Autodesk Inventor part; units mm, degrees
ref_plane "YZ Plane" through (0, 0, 0) normal (1, 0, 0) x (0, 1, 0)
ref_plane "XZ Plane" through (0, 0, 0) normal (0, 1, 0) x (-1, 0, 0)
ref_plane "XY Plane" through (0, 0, 0) normal (0, 0, 1) x (1, 0, 0)
sketch "Sketch1" plane through (0, 0, 0) normal (0, 0, 1) x (1, 0, 0)
  circle A0 centre (0, 0) radius 4
  arc A1 (-6, 0) -> (6, 0) centre (0, 0) ccw
  line L0 (0, 21) -> (13.5, 21)
  line L1 (13.5, 21) -> (-13.5, 21)
  line L2 (-13.5, 21) -> (-13.5, 12)
  line L3 (-13.5, 12) -> (-6, 0)
  line L4 (13.5, 21) -> (13.5, 12)
  line L5 (13.5, 12) -> (6, 0)
  dimension "d0" = 8
  dimension "d1" = 12
  dimension "d2" = 21
  dimension "d3" = 13.5
  dimension "d4" = 27
  dimension "d5" = 9
  dimension "d6" = 9
extrude "Extrusion1" add sketch "Sketch1" along normal blind 3
sketch "Sketch2" plane through (13.5, 12, 0) normal (1, 0, 0) x (0, 0, -1)
  line L0 (8, 20) -> (-3, 9)
  line L1 (8, 20) -> (68, 20)
  line L2 (79, 9) -> (68, 20)
  line L3 (0, 9) -> (-3, 9)
  line L4 (-3, 9) -> (0, 9)
  line L5 (0, 9) -> (8, 17)
  line L6 (79.1439, 8.8561) -> (76.1439, 8.8561)
  line L7 (76.1439, 8.8561) -> (68, 17)
  line L8 (39.224, 17) -> (8, 17)
  line L9 (39.224, 17) -> (68, 17)
  line L10 (-3, 0) -> (-3, -12)
  line L11 (8, 17) -> (68, 17)
  line L12 (-3, 9) -> (0, 9)
  line L13 (0, 9) -> (8, 17)
  line L14 (8, 17) -> (68, 17)
  line L15 (76.1439, 8.8561) -> (79.1439, 8.8561)
  line L16 (79.1439, 8.8561) -> (68, 20)
  line L17 (68, 20) -> (8, 20)
  line L18 (8, 20) -> (-3, 9)
  line L19 (-3, 9) -> (0, 9)
  point P0 (0, -12)
  dimension "d11" = 60
  dimension "d14" = 3
extrude "Extrusion2" add sketch "Sketch2" against normal blind 27
sketch "Sketch3" plane through (13.5, 20.8561, -79.1439) normal (0, -1, 0) x (1, 0, 0)
  line L0 (0, 0) -> (-27, 0)
  line L1 (0, 0) -> (-27, 0)
  line L2 (0, 3) -> (-27, 3)
  line L3 (-27, 0) -> (-27, 3)
  line L4 (-27, 3) -> (0, 3)
  line L5 (0, 3) -> (0, 0)
  point P0 (-13.5, 79.1439)
extrude "Extrusion3" add sketch "Sketch3" along normal blind 45
sketch "Sketch4" plane through (13.5, 29, -68) normal (0, -1, 0) x (1, 0, 0)
  line L0 (0, 0) -> (0, 60)
  line L1 (0, 1.254) -> (-27, 1.254)
  line L2 (-27, 0) -> (-27, 60)
  line L3 (0, 1.254) -> (-13.5, 1.254)
  line L4 (-13.5, 1.254) -> (4, 1.254)
  line L5 (4, 1.254) -> (4, 49.254)
  line L6 (4, 49.254) -> (-31, 49.254)
  line L7 (-31, 49.254) -> (-31, 1.254)
  line L8 (-31, 1.254) -> (4, 1.254)
  point P0 (-13.5, 68)
  dimension "d20" = 1.254
  dimension "d21" = 17.5
  dimension "d22" = 48
  dimension "d23" = 35
extrude "Extrusion4" add sketch "Sketch4" along normal blind 26
sketch "Sketch5" plane through (13.5, 32, -8) normal (0, 1, 0) x (1, 0, 0)
  line L0 (-27, 0) -> (-27, 60)
  line L1 (0, 60) -> (-27, 60)
  circle A0 centre (-13.5, 46.746) radius 4
  point P0 (-13.5, -8)
  dimension "d28" = 8
extrude "Extrusion5" add sketch "Sketch5" along normal blind 10
sketch "Sketch6" plane through (13.5, 20.8561, -79.1439) normal (0, 0, -1) x (-1, 0, 0)
  circle A0 centre (13.5, -21) radius 4
  arc A1 (7.5004, -20.9281) -> (19.4996, -20.9281) centre (13.5, -21) ccw
  line L0 (27, -9) -> (19.5, -21)
  line L1 (7.5, -20.8561) -> (0, -8.8561)
  line L2 (0, -8.8561) -> (7.5, -20.8561)
  line L3 (27, 0) -> (27, -45)
  line L4 (27, -9) -> (27, -45)
  line L5 (0, -45) -> (27, -45)
  line L6 (27, -45) -> (0, -45)
  line L7 (0, -45) -> (0, -8.8561)
  arc A2 (7.5, -20.8561) -> (19.5, -20.8561) centre (13.5, -20.8561) ccw
  arc A3 (7.5, -20.8561) -> (19.5, -20.8561) centre (13.5, -21) ccw
  point P0 (0, 0.1439)
  dimension "d34" = 8
  dimension "d35" = 12
extrude "Extrusion6" cut sketch "Sketch6" against normal blind 4 contours A0 | A1 L0 L3 L5 L7 L1 A2
properties part number "Cversion2"
Geometry check sheet. Reference: the model listing, model coordinates, mm. A direction names the side the tool comes from. Coordinates: 2 decimals unless noted, no trailing zeros. Write each loop counter-clockwise with the first axis right and the second up, starting at its lowest first coordinate (ties: lowest second). Pieces come first, ordered by that corner, then holes. Notation, with made-up numbers: M 33.5,-23.5 L 85.5,-23.5 A19 cw 85.5,-16.5 Z; hole C -1.75,74.5 d8. An arc over 180 degrees is marked long. Use one line per item in the form item = value. Start each with the question number.
1) Thickness scan on probe 1 along Z at (x, y) = (-2.5, 10); probe 2 along Z at (x, y) = (0.5, 28); probe 3 along Y at (x, z) = (-6, -24). Record the ranges inside material, lowest first. Write a range as from..to.
2) Release check for a two-part mould opening along Z. For faces 1 (the flat face through (0, 26, -74)), 2 (the flat face through (0, 29, -13)), 3 (the flat face through (0, 11, 3)) record: pulls with the +Z half, pulls with the -Z half, needs draft (parallel to the pull), parting line crosses it, or undercut.
3) Section check D-D on y = -1. Enter the section's corners in (x, z).
4) Section check A-A on y = 19. Enter the section's corners in (x, z), and give its area (3 significant figures).
5) Set-up check for faces 4 (the cylindrical face through (-0.867, 3.905, 1.479)), 5 (the cylindrical face through (0, -6, 1)), 6 (the flat face through (-16, 29, -42)), 7 (the flat face through (0, 3, -42)): record each of +Z, -Z, +X, -X, +Y, -Y from which the full face is reachable in a straight line by a thin tool's end or side.
6) Go/stop test with flat-tipped pins: pin 1 Ø12 at (x, z) = (-6, -12.5) entering from -Y; pin 2 Ø3 at (x, z) = (-16, -42.5) entering from +Y; pin 3 Ø0.6 at (x, z) = (-5, -67.5) entering from -Y. Record where each tip stops, or that it passes through.
7) Section check C-C on z = -31. Enter the section's corners in (x, y).
8) Section check B-B on x = 1. Enter the section's corners in (y, z).
Responses:
q1.probe_1 = -79.14..-76.14, -66.75..-18.75, 0..3
q1.probe_2 = -72..-69, -66.75..-18.75, -7..-4
q1.probe_3 = 3..32
q2.face_1 = pulls with the -Z half
q2.face_2 = undercut
q2.face_3 = pulls with the +Z half
q3.outline = M -5.94,-79.14 L -3.91,-79.14 L -3.91,-76.14 L -5.94,-76.14 Z; M -5.92,0 L -3.87,0 L -3.87,3 L -5.92,3 Z; M 3.87,0 L 5.92,0 L 5.92,3 L 3.87,3 Z; M 3.91,-79.14 L 5.94,-79.14 L 5.94,-76.14 L 3.91,-76.14 Z
q4.outline = M -17.5,-66.75 L 17.5,-66.75 L 17.5,-18.75 L -17.5,-18.75 Z; M -13.5,-79.14 L 13.5,-79.14 L 13.5,-76.14 L -13.5,-76.14 Z; M -13.5,0 L 13.5,0 L 13.5,3 L -13.5,3 Z
q4.area = 1,840 mm2
q5.face_4 = +Z
q5.face_5 = +Z, -Y
q5.face_6 = +Z, -Z, -X, +Y
q5.face_7 = +X, -X, -Y
q6.pin_1 = 27.5
q6.pin_2 = 29
q6.pin_3 = 29
q7.outline = M -17.5,3 L 17.5,3 L 17.5,29 L 13.5,29 L 13.5,32 L -13.5,32 L -13.5,29 L -17.5,29 Z
q8.outline = M -6.06,-79.14 L -4.02,-79.14 L -4.02,-76.14 L -6.06,-76.14 Z; M -5.92,0 L -3.87,0 L -3.87,3 L -5.92,3 Z; M 3,-66.75 L 29,-66.75 L 29,-68 L 20.86,-76.14 L 3.73,-76.14 L 3.73,-79.14 L 20.86,-79.14 L 32,-68 L 32,-58.62 L 42,-58.62 L 42,-50.87 L 32,-50.87 L 32,-8 L 21,3 L 3.87,3 L 3.87,0 L 21,0 L 29,-8 L 29,-18.75 L 3,-18.75 Z
